```python
from build123d import *

# Parameters (mm, degrees)
F0_W     = 20
F0_H     = 50
F1_DEPTH = 20
F2_R     = 0.508
F3_R     = 2.5
F4_DEPTH = 70
F5_W     = 12
F5_H     = 40
F5_R     = 2.5
F6_DEPTH = 10


# Not quite as in the source:
# - a feature names something its author has since deleted; it is built from what else it names


with BuildPart() as f1:
    # F0 (on Front) → F1 (new body)
    with BuildSketch(Plane.XZ):
        with Locations((0, 15)):
            Rectangle(F0_W, F0_H)
    extrude(amount=F1_DEPTH)

    # F2
    f2_edges = [f1.edges().sort_by_distance(p)[0] for p in [
        (0, -20, 40),
        (-10, -20, 15),
        (0, -20, -10),
        (10, -20, 15),
        (10, -10, -10),
        (10, -10, 40),
        (10, 0, 15),
        (-10, -10, 40),
        (0, 0, 40),
        (-10, -10, -10),
        (-10, 0, 15),
        (0, 0, -10),
    ]]
    fillet(f2_edges, radius=F2_R)

    # F3 (on face) → F4 (join)
    with BuildSketch(Plane.XZ.offset(20)):
        with Locations((0, 30)):
            Circle(F3_R)
        Circle(F3_R)
    extrude(amount=F4_DEPTH)

    # F5 (on face) → F6 (join)
    with BuildSketch(Plane.XZ.offset(90)):
        with Locations((0, 15)):
            Rectangle(F5_W, F5_H)
        with Locations((0, 30)):
            Circle(F5_R, mode=Mode.SUBTRACT)
        with Locations((0, 30)):
            Circle(F5_R)
    extrude(amount=F6_DEPTH)


solid = f1.part
```
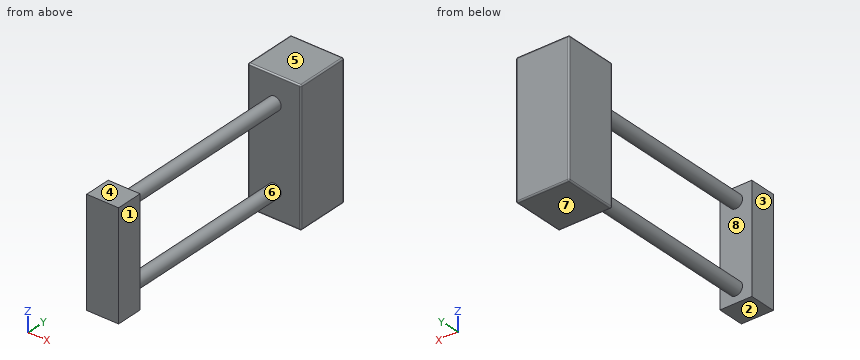
CAD build for the part. Positions are in the model's coordinates, mm. Face numbers are marked on the shaded views. A direction names the side the tool comes from. Give positions to 0.01 mm unless a question says otherwise; leave off trailing zeros. Write each loop counter-clockwise with the first axis right and the second up, starting at its lowest first coordinate (ties: lowest second). Pieces come first, ordered by that corner, then holes. Notation, with made-up numbers: M -26,9.5 L -18,9.5 A22 cw -18,48.5 Z; hole C -7,34 d3. An arc over 180 degrees is marked long. Return JSON: item names as keys, results as strings. Group by question number.
(1) Band-saw the part on D-D (x = 0). Give the cut face in (y, z), and give its area (3 significant figures).
(2) Band-saw the part on B-B (x = 4.25). Give the cut face in (y, z).
(3) 3-axis set-ups, long thin cutter, end or side, ignore diameter. For the marked faces 1, 2, 3 and 4: which of +Z, -Z, +X, -X, +Y, -Y reach the whole face in a straight line?
(4) Band-saw the part on A-A (z = 25). Give the cut face in (x, y), and give its area (3 significant figures).
(5) Mould opens along Z. For the marked faces 5, 6, 7 and 8 say: pulls with the +Z half, pulls with the -Z half, needs draft (parallel to the pull), parting line crosses it, or undercut.
(6) Band-saw the part on C-C (y = -28.5). Give the cut face in (x, z).
(7) Drill centre lines: L1, parallel to Y at x = -1.25, z = -4; L2, parallel to Z at x = 0, y = -85; L3, parallel to Y at x = 7, z = 33. Where is each one in solid material? Low to high. Write a range as [from, to].
(8) Flat gauge pins, fed straight in: pin 1 Ø8 at (x, y) = (2, -49) entering from -Z; pin 2 Ø5 at (y, z) = (-30.5, -4) entering from +X; pin 3 Ø8 at (x, y) = (2, -93) entering from -Z; pin 4 Ø1 at (y, z) = (-27.5, 4) entering from -X. Where does each tip first touch, or does it go through?
Entries:
{
 "1": {"outline": "M -100,-5 L -90,-5 L -90,-2.5 L -20,-2.5 L -20,-9.49 A0.51 ccw -19.49,-10 L -0.51,-10 A0.51 ccw 0,-9.49 L 0,39.49 A0.51 ccw -0.51,40 L -19.49,40 A0.51 ccw -20,39.49 L -20,32.5 L -90,32.5 L -90,35 L -100,35 Z; hole M -90,2.5 L -20,2.5 L -20,27.5 L -90,27.5 Z", "area": "2,100 mm^2"},
 "2": {"outline": "M -100,-5 L -90,-5 L -90,35 L -100,35 Z; M -20,-9.49 A0.51 ccw -19.49,-10 L -0.51,-10 A0.51 ccw 0,-9.49 L 0,39.49 A0.51 ccw -0.51,40 L -19.49,40 A0.51 ccw -20,39.49 Z"},
 "3": {"face 1": "+Z, -Z, +X, -Y", "face 2": "-Z, +X, -X, -Y", "face 3": "+Z, -Z, -X, -Y", "face 4": "+Z, +X, -X, -Y"},
 "4": {"outline": "M -10,-19.49 A0.51 ccw -9.49,-20 L 9.49,-20 A0.51 ccw 10,-19.49 L 10,-0.51 A0.51 ccw 9.49,0 L -9.49,0 A0.51 ccw -10,-0.51 Z; M -6,-100 L 6,-100 L 6,-90 L -6,-90 Z", "area": "520 mm^2"},
 "5": {"face 5": "pulls with the +Z half", "face 6": "undercut", "face 7": "pulls with the -Z half", "face 8": "undercut"},
 "6": {"outline": "C 0,0 d5; C 0,30 d5"},
 "7": {"L1": "y = [-100, -90], [-20, 0]", "L2": "z = [-2.5, 2.5], [27.5, 32.5]", "L3": "y = [-20, 0]"},
 "8": {"pin 1": "stops at z = -2.5", "pin 2": "stops at x = 2", "pin 3": "stops at z = -5", "pin 4": "passes through"}
}
